Input: dimensioned drawing with shaded views. Units: mm. Origin: part minimum x, y, z. A direction names the side the tool comes from. Coordinates: 2 decimals unless noted, no trailing zeros. Order: outer loops, then holes, each group sorted by start corner. A loop starts at its lowest first (then second) coordinate and runs counter-clockwise, first axis right, second up. Notation, with made-up numbers: (79.5, -18.75) -> (101.5, -18.75) arc R8 cw to (101.5, -14.75) -> close; hole circle Ø3 at (42.25, -20.75). An arc over 180 degrees is marked (long way). Answer as CSV lines item,"result".
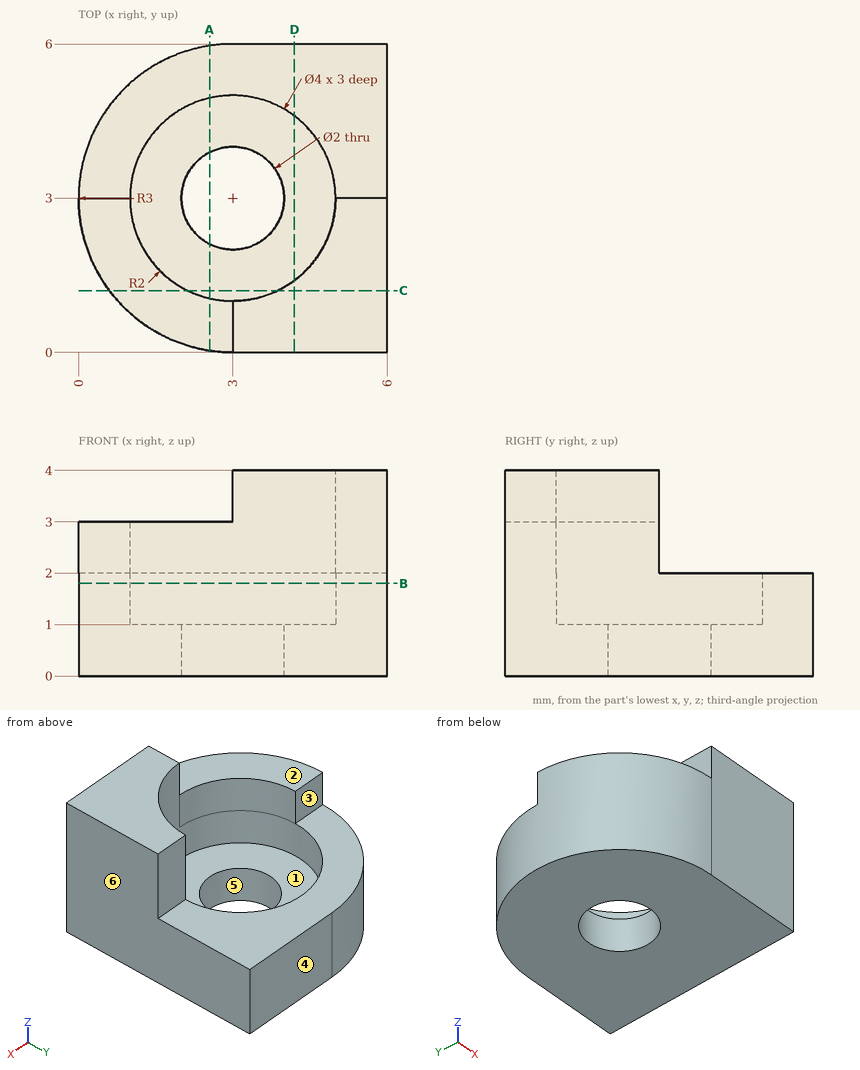
1. Cut plane A-A (x = 2.55). Return the cut outline in (y, z), plus the area to 3 significant figures.
Findings:
outline,"(0.03, 0) -> (2.11, 0) -> (2.11, 1) -> (1.05, 1) -> (1.05, 3) -> (0.03, 3) -> close; (3.89, 0) -> (5.97, 0) -> (5.97, 2) -> (4.95, 2) -> (4.95, 1) -> (3.89, 1) -> close"
area,"7.20 mm2"
2. Cut plane D-D (x = 4.2). Return the cut outline in (y, z).
Findings:
outline,"(0, 0) -> (6, 0) -> (6, 2) -> (4.6, 2) -> (4.6, 1) -> (1.4, 1) -> (1.4, 4) -> (0, 4) -> close"
3. Mould query, pull axis Y, two halves, no side actions, for the marked faces 4, 5 and 6. Classes: released by +Y, released by -Y, zero draft, split by the parting line, or undercut.
Findings:
face 4,"released by +Y"
face 5,"undercut"
face 6,"zero draft"
4. Cut plane C-C (y = 1.2). Return the cut outline in (x, z).
Findings:
outline,"(0.6, 0) -> (6, 0) -> (6, 4) -> (3.87, 4) -> (3.87, 1) -> (2.13, 1) -> (2.13, 3) -> (0.6, 3) -> close"
5. Contact query for flat-ended pins moving along their axis: pin 1 (0.5 mm diameter, centred on y = 0.5, z = 3.5, fed in from -X); pin 2 (0.9 mm diameter, centred on x = 1.5, y = 2, fed in from +Z); pin 3 (0.5 mm diameter, centred on x = 0.5, z = 2.5, fed in from +Y). Output: stop coordinate, or through.
Findings:
pin 1,"stops at x = 3"
pin 2,"stops at z = 3"
pin 3,"stops at y = 3"
6. Reachability of the marked faces 1, 2 and 3 from +Z, -Z, +X, -X, +Y, -Y: full face, straight path, thin tool, end or side. Return the list, or none.
Findings:
face 1,"+Z"
face 2,"+Z, -X, +Y, -Y"
face 3,"+Z, +X, -X, +Y"
7. Ray query, line 1 along Y through (x, z) = (3, 0.45); line 2 along Z through (x, y) = (4, 5.4); line 3 along X through (y, z) = (0.45, 3.55). Return the intervals inside material, ascending.
Findings:
line 1,"y = 0 to 2, 4 to 6"
line 2,"z = 0 to 2"
line 3,"x = 3 to 6"
8. Cut plane B-B (z = 1.8). Return the cut outline in (x, y), plus the area to 3 significant figures.
Findings:
outline,"(3, 0) -> (6, 0) -> (6, 6) -> (3, 6) arc R3 ccw to start; hole circle Ø4 at (3, 3)"
area,"19.6 mm2"
